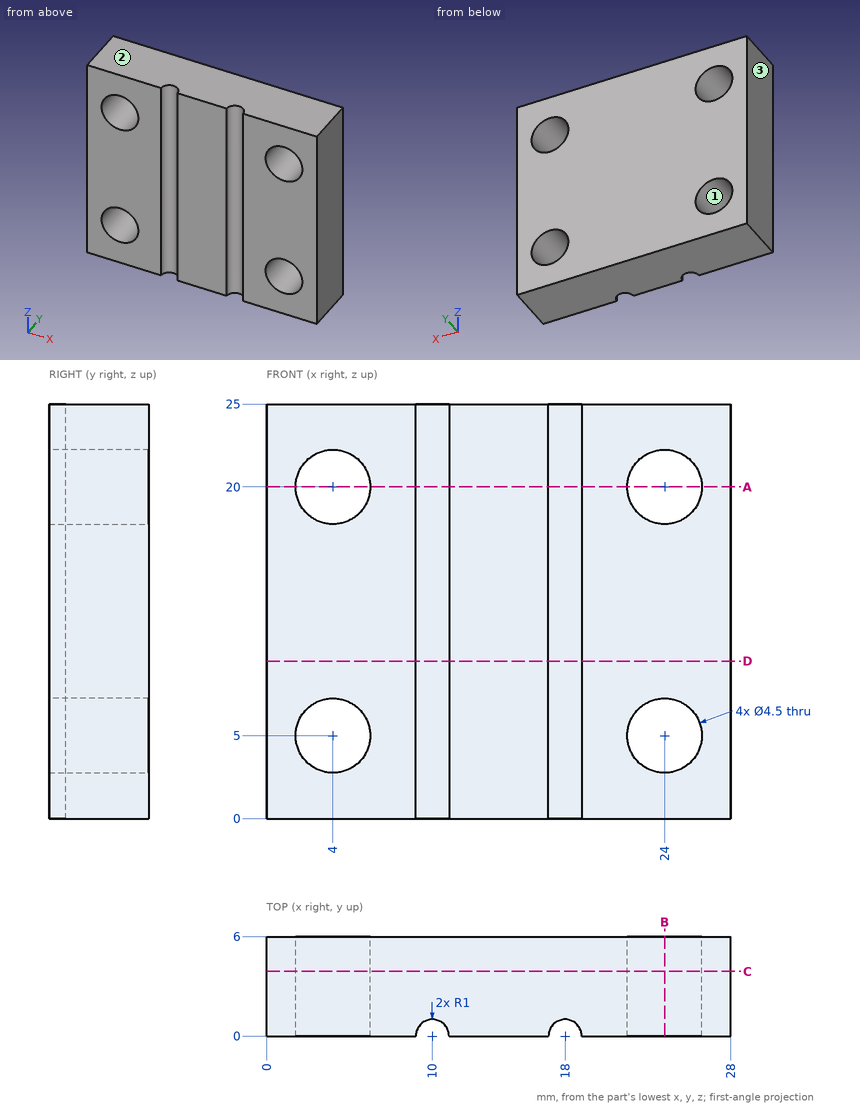
Check sheet for the drawn part. Datum: minimum x, y, z corner. Units: mm. Round coordinates to 2 decimals unless told otherwise and drop trailing zeros. Write each loop counter-clockwise with the first axis right and the second up, starting at its lowest first coordinate (ties: lowest second). Pieces come first, ordered by that corner, then holes. Notation, with made-up numbers: (56.25, -27) -> (61.25, -27) arc R29 cw to (61.25, 8) -> close; hole circle Ø10 at (12.25, 87.25). An arc over 180 degrees is marked (long way). Put each result on its own line as item: value.
(1) Sectioned sample at C-C (y = 3.9). Enter the section's corners in (x, z), plus the area to 3 significant figures.
Values found:
outline: (0, 0) -> (28, 0) -> (28, 25) -> (0, 25) -> close; hole circle Ø4.5 at (4, 5); hole circle Ø4.5 at (4, 20); hole circle Ø4.5 at (24, 5); hole circle Ø4.5 at (24, 20)
area: 636 mm^2
(2) Material ranges on line 1 (X direction, y = 3.9, z = 20); line 2 (Z direction, x = 23.5, y = 1.1); line 3 (X direction, y = 3.75, z = 19), recorded low to high.
Values found:
line 1: x = 0 to 1.75, 6.25 to 21.75, 26.25 to 28
line 2: z = 0 to 2.81, 7.19 to 17.81, 22.19 to 25
line 3: x = 0 to 1.98, 6.02 to 21.98, 26.02 to 28
(3) Sectioned sample at A-A (z = 20). Enter the section's corners in (x, y), plus the area to 3 significant figures.
Values found:
outline: (0, 0) -> (1.75, 0) -> (1.75, 6) -> (0, 6) -> close; (6.25, 0) -> (9, 0) arc R1 cw to (11, 0) -> (17, 0) arc R1 cw to (19, 0) -> (21.75, 0) -> (21.75, 6) -> (6.25, 6) -> close; (26.25, 0) -> (28, 0) -> (28, 6) -> (26.25, 6) -> close
area: 111 mm^2
(4) Sectioned sample at D-D (z = 9.5). Enter the section's corners in (x, y), plus the area to 3 significant figures.
Values found:
outline: (0, 0) -> (9, 0) arc R1 cw to (11, 0) -> (17, 0) arc R1 cw to (19, 0) -> (28, 0) -> (28, 6) -> (0, 6) -> close
area: 165 mm^2
(5) Sectioned sample at B-B (x = 24). Enter the section's corners in (y, z).
Values found:
outline: (0, 0) -> (6, 0) -> (6, 2.75) -> (0, 2.75) -> close; (0, 7.25) -> (6, 7.25) -> (6, 17.75) -> (0, 17.75) -> close; (0, 22.25) -> (6, 22.25) -> (6, 25) -> (0, 25) -> close
(6) Mould release check, pull along X, two halves, no side actions. Record for the marked faces 1, 2 and 3: released by +X, released by -X, zero draft, split by the parting line, or undercut.
Values found:
face 1: undercut
face 2: zero draft
face 3: released by -X
